Model file for the job. Use its own axes, mm. Face numbers are marked on the shaded views. A direction names the side the tool comes from. Give positions to 0.01 mm unless a question says otherwise; leave off trailing zeros. Write each loop counter-clockwise with the first axis right and the second up, starting at its lowest first coordinate (ties: lowest second). Pieces come first, ordered by that corner, then holes.
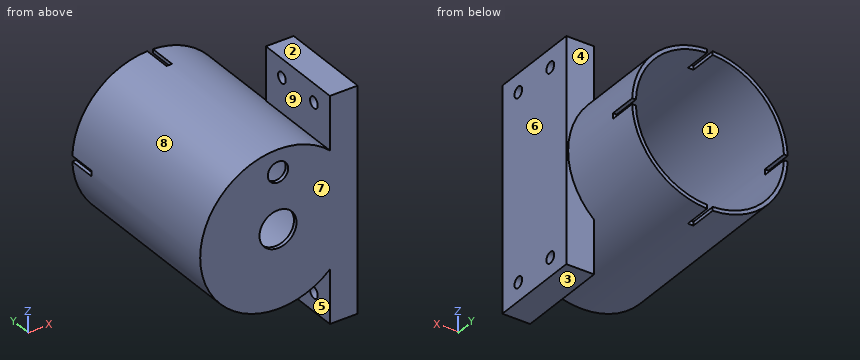
```python
from build123d import *

# Parameters (mm, degrees)
ESBO_O1_R                = 42
RESSALTO_EXTRUS_O1_DEPTH = 100
ESBO_O2_R                = 40
CORTE_EXTRUS_O1_DEPTH    = 98
ESBO_O3_R                = 5.5
CORTE_EXTRUS_O2_DEPTH    = 117.309930788
ESBO_O4_R                = 10
CORTE_EXTRUS_O3_DEPTH    = 117.309930788
CORTE_EXTRUS_O4_DEPTH    = 15
RESSALTO_EXTRUS_O3_DEPTH = 50
ESBO_O9_R                = 3
CORTE_EXTRUS_O5_DEPTH    = 137.014705087


with BuildPart() as part:
    # Esboço1 → Ressalto-extrusão1 (new body)
    with BuildSketch(Plane(origin=(0, 0, 0), x_dir=(1, 0, 0), z_dir=(0, 1, 0))):
        with Locations(Location((0, 0, 0), (0, 0, 270))):
            Circle(ESBO_O1_R)
    extrude(amount=RESSALTO_EXTRUS_O1_DEPTH)

    # Esboço2 → Corte-extrusão1 (cut)
    with BuildSketch(Plane(origin=(0, 100, 0), x_dir=(1, 0, 0), z_dir=(0, 1, 0))):
        with Locations(Location((0, 0, 0), (0, 0, 270))):
            Circle(ESBO_O2_R)
    extrude(amount=-CORTE_EXTRUS_O1_DEPTH, mode=Mode.SUBTRACT)

    # Esboço3 → Corte-extrusão2 (cut, through all)
    with BuildSketch(Plane.XZ):
        with Locations(Location((0, 30, 0), (0, 0, 270))):
            Circle(ESBO_O3_R)
    extrude(amount=-CORTE_EXTRUS_O2_DEPTH, mode=Mode.SUBTRACT)

    # Esboço4 → Corte-extrusão3 (cut, through all)
    with BuildSketch(Plane.XZ):
        with Locations(Location((0, 0, 0), (0, 0, 270))):
            Circle(ESBO_O4_R)
    extrude(amount=-CORTE_EXTRUS_O3_DEPTH, mode=Mode.SUBTRACT)

    # Esboço5 → Corte-extrusão4 (cut)
    with BuildSketch(Plane(origin=(0, 100, 0), x_dir=(1, 0, 0), z_dir=(0, 1, 0))):
        Polygon((1.5, 1.5), (52.94033898, 1.5), (52.94033898, -1.5), (1.5, -1.5), (1.5, -46.298898587), (-1.5, -46.298898587), (-1.5, -1.5), (-52.94033898, -1.5), (-52.94033898, 1.5), (-1.5, 1.5), (-1.5, 46.298898587), (1.5, 46.298898587), align=None)
    extrude(amount=-CORTE_EXTRUS_O4_DEPTH, mode=Mode.SUBTRACT)

    # Esboço8 → Ressalto-extrusão3 (add)
    with BuildSketch(Plane.XZ):
        with BuildLine():
            Line((28, 31.304951685), (28, 60))
            Line((28, 60), (43, 60))
            Line((43, 60), (43, -60))
            Line((43, -60), (28, -60))
            Line((28, -60), (28, -31.304951685))
            ThreePointArc((28, -31.304951685), (42, 0), (28, 31.304951685))
        make_face()
    extrude(amount=-RESSALTO_EXTRUS_O3_DEPTH)

    # Esboço9 → Corte-extrusão5 (cut, through all)
    with BuildSketch(Plane.ZY.offset(-28)):
        with Locations((50, 37.5)):
            Circle(ESBO_O9_R)
        with Locations((50, 12.5)):
            Circle(ESBO_O9_R)
        with Locations(Location((-50, 12.5, 0), (0, 0, 180))):
            Circle(ESBO_O9_R)
        with Locations(Location((-50, 37.5, 0), (0, 0, 180))):
            Circle(ESBO_O9_R)
    extrude(amount=-CORTE_EXTRUS_O5_DEPTH, mode=Mode.SUBTRACT)


solid = part.part
```
1. Pull direction X, two halves, no side cores. Call the marked faces 6, 7, 8 and 9: +X half, -X half, draft (parallel to the pull), parting line (faces both ways), or undercut.
Calculated:
face 6: +X half
face 7: draft
face 8: undercut
face 9: undercut
2. Slice it at D-D, the plane z = 50. Write the cut outline in (x, y).
Calculated:
outline: (28, 0) - (43, 0) - (43, 9.5) - (28, 9.5) - close; (28, 15.5) - (43, 15.5) - (43, 34.5) - (28, 34.5) - close; (28, 40.5) - (43, 40.5) - (43, 50) - (28, 50) - close
3. Slice it at A-A, the plane y = 12.5. Write the cut outline in (x, z), and give its area (3 significant figures).
Calculated:
outline: (28, -60) - (43, -60) - (43, -53) - (28, -53) - close; (28, -47) - (43, -47) - (43, 47) - (28, 47) - (28, 31.3) arc R42 ccw (long way) to (28, -31.3) - close; (28, 53) - (43, 53) - (43, 60) - (28, 60) - close; hole circle Ø80 at (0, 0)
area: 1,530 mm2
4. Slice it at B-B, the plane x = 0. Write the cut outline in (y, z).
Calculated:
outline: (0, -42) - (85, -42) - (85, -40) - (2, -40) - (2, -10) - (0, -10) - close; (0, 10) - (2, 10) - (2, 24.5) - (0, 24.5) - close; (0, 35.5) - (2, 35.5) - (2, 40) - (85, 40) - (85, 42) - (0, 42) - close
5. Slice it at C-C, the plane z = 0. Write the cut outline in (x, y).
Calculated:
outline: (-42, 0) - (-10, 0) - (-10, 2) - (-40, 2) - (-40, 85) - (-42, 85) - close; (10, 0) - (43, 0) - (43, 50) - (42, 50) - (42, 85) - (40, 85) - (40, 2) - (10, 2) - close
6. Pin check, flat tips, straight feed: P1, Ø6, axis at x = 0, y = 15.5, coming from the -Z side; P2, Ø5, axis at y = 87.5, z = 33.5, coming from the +X side; P3, Ø1.6, axis at x = 0.5, z = -40.5, coming from the +Y side; P4, Ø18, axis at x = 0, z = 0, coming from the +Y side. Stop position of each tip, or through.
Calculated:
P1: stops at z = -42
P2: stops at x = 28.34
P3: stops at y = 85
P4: passes through
7. Which spindle directions (+Z, -Z, +X, -X, +Y, -Y) get a long thin tool onto all of the face, cutting with end or side? Do the marked faces 1, 2, 3, 4 and 5. Say none if no direction does.
Calculated:
face 1: +Y
face 2: +Z, +X, -X, +Y, -Y
face 3: -Z, +X, -X, +Y, -Y
face 4: +X, +Y
face 5: -Z, +Y, -Y
8. Probe probe 1 along Y at (x, z) = (35.75, -50); probe 2 along Z at (x, y) = (0, 32); probe 3 along X at (y, z) = (1, 0). List the from-to ranges inside material, lowest first.
Calculated:
probe 1: y = 0 to 9.5, 15.5 to 34.5, 40.5 to 50
probe 2: z = -42 to -40, 40 to 42
probe 3: x = -42 to -10, 10 to 43
